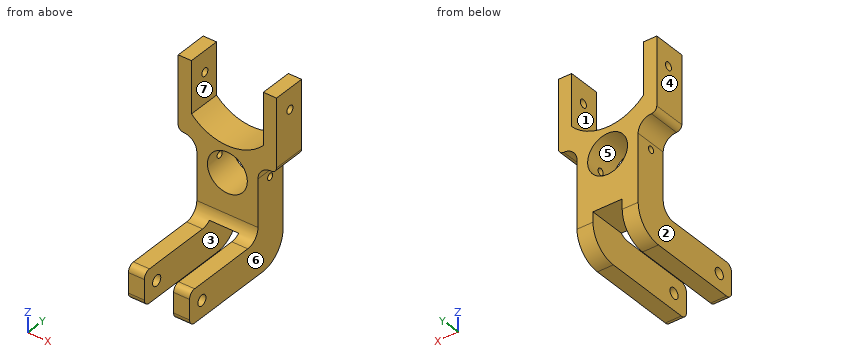
```python
from build123d import *

# Parameters (mm, degrees)
EXTRUDE_START         = -3
EXTRUDE_1_DEPTH       = 46
SKETCH_2_R            = 15
SKETCH_2_W            = 22
SKETCH_2_H            = 41.003909118
CUT_EXTRUDE_2_DEPTH   = 120
SKETCH_3_R            = 4
SKETCH_3_R_2          = 2.5
CUT_EXTRUDE_1_DEPTH   = 55
SKETCH_4_W            = 74
SKETCH_4_H            = 24.59688775
EXTRUDE_3_DEPTH       = 55
CUT_EXTRUDE_2_2_DEPTH = 50
FILLET_2_R            = 4
SKETCH_7_R            = 3
CUT_EXTRUDE_3_DEPTH   = 90
FILLET_3_R            = 10


with BuildPart() as part:
    # Эскиз1 → Вытянуть1 (new body)
    with BuildSketch(Plane(origin=(0, 0, 0), x_dir=(0, 0, -1), z_dir=(1, 0, 0)).offset(EXTRUDE_START)):
        with BuildLine():
            Line((3.683652722, 0), (3.683652722, -24.59688775))
            Line((3.683652722, -24.59688775), (49.132150834, -24.59688775))
            ThreePointArc((49.132150834, -24.59688775), (56.203219269, -27.52582056), (59.132150834, -34.59688951))
            Line((59.132150834, -34.59688951), (59.132141638, -86.831595085))
            ThreePointArc((59.132141638, -86.831595085), (60.596607421, -90.36712956), (64.132141638, -91.831595966))
            Line((64.132141638, -91.831595966), (79.132150834, -91.831595966))
            ThreePointArc((79.132150834, -91.831595966), (82.66768474, -90.367129871), (84.132150834, -86.831595966))
            Line((84.132150834, -86.831595966), (84.132150834, -20))
            ThreePointArc((84.132150834, -20), (78.274286458, -5.857864376), (64.132150834, 0))
            Line((64.132150834, 0), (3.683652722, 0))
        make_face()
    extrude(amount=EXTRUDE_1_DEPTH)

    # Эскиз2 → Cut-Extrude 2 (cut, symmetric)
    with BuildSketch(Plane(origin=(0, 0, 0), x_dir=(1, 0, 0), z_dir=(0, 1, 0))):
        with Locations(Location((20, 18.931682227, 0), (0, 0, 270))):
            Circle(SKETCH_2_R)
        with Locations((20, 77.079487522)):
            Rectangle(SKETCH_2_W, SKETCH_2_H)
    extrude(amount=CUT_EXTRUDE_2_DEPTH, both=True, mode=Mode.SUBTRACT)

    # Эскиз3 → Вырез-Вытянуть1 (cut, symmetric)
    with BuildSketch(Plane(origin=(0, 0, 0), x_dir=(0, 0, -1), z_dir=(1, 0, 0))):
        with Locations((71.632122158, -79.695359499)):
            Circle(SKETCH_3_R)
        with Locations((18.675004926, -12.628238718)):
            Circle(SKETCH_3_R_2)
    extrude(amount=CUT_EXTRUDE_1_DEPTH, both=True, mode=Mode.SUBTRACT)

    # Эскиз4 → Вытянуть3 (add)
    with BuildSketch(Plane.XY.offset(-3.683652722)):
        with Locations((20.003387868, -12.298443875)):
            Rectangle(SKETCH_4_W, SKETCH_4_H)
    extrude(amount=EXTRUDE_3_DEPTH)

    # Эскиз6 → Cut-Extrude 2 2 (cut, symmetric)
    with BuildSketch(Plane(origin=(0, 0, 0), x_dir=(1, 0, 0), z_dir=(0, 1, 0))):
        with BuildLine():
            Line((47.003387868, -53.712819086), (47.003387868, -12.467045061))
            ThreePointArc((47.003387868, -12.467045061), (20.003387863, -0.765266352), (-6.996612132, -12.467045083))
            Line((-6.996612132, -12.467045083), (-6.996612132, -53.712819086))
            Line((-6.996612132, -53.712819086), (47.003387868, -53.712819086))
        make_face()
    extrude(amount=CUT_EXTRUDE_2_2_DEPTH, both=True, mode=Mode.SUBTRACT)

    # Скругление2
    fillet_2_edges = [part.edges().sort_by_distance(p)[0] for p in [
        (57.003387868, -12.298443875, -3.683652722),
        (-16.996612132, -12.298443875, -3.683652722),
    ]]
    fillet(fillet_2_edges, radius=FILLET_2_R)

    # Эскиз7 → Вырез-Вытянуть3 (cut, symmetric)
    with BuildSketch(Plane(origin=(57.003387868, 0, 0), x_dir=(0, 0, -1), z_dir=(1, 0, 0))):
        with Locations((-35.623538585, -11.460561108)):
            Circle(SKETCH_7_R)
    extrude(amount=CUT_EXTRUDE_3_DEPTH, both=True, mode=Mode.SUBTRACT)

    # Скругление3
    fillet_3_edges = [part.edges().sort_by_distance(p)[0] for p in [
        (-3, -12.298443875, -3.683652722),
        (43, -12.298443875, -3.683652722),
    ]]
    fillet(fillet_3_edges, radius=FILLET_3_R)


solid = part.part
```
Geometry check sheet. Reference: the model listing, model coordinates, mm. Face numbers are marked on the shaded views. A direction names the side the tool comes from. Coordinates: 2 decimals unless noted, no trailing zeros. Order: outer loops, then holes, each group sorted by start corner. A loop starts at its lowest first (then second) coordinate and runs counter-clockwise, first axis right, second up. Notation, with made-up numbers: (-9.5, 15.25) - (34.5, 15.25) arc R21 ccw to (34.5, 46.25) - close; hole circle Ø8 at (61.5, -23). An arc over 180 degrees is marked (long way). Answer as a JSON object with one key per item and string values. Group by question number.
Item 1: Depth check by flat-ended pin: pin 1 Ø2 at (x, z) = (25, -43.5) entering from -Y; pin 2 Ø13 at (x, y) = (35.5, -71) entering from +Z; pin 3 Ø6 at (y, z) = (-79, -64.5) entering from +X. Enter the tip coordinate at first touch or a pass-through.
Item 2: Sectioned sample at B-B, the plane y = -60. Record the cut outline in (x, z), and give its area (3 significant figures).
Item 3: Draft check along X on the marked faces 4, 5, 6 and 7. Enter one of: +X half, -X half, draft (parallel to the pull), parting line (faces both ways), or undercut.
Item 4: Sectioned sample at C-C, the plane z = 15.5. Record the cut outline in (x, y).
Item 5: Scan lines: probe 1 along X at (y, z) = (-7, -76); probe 2 along X at (y, z) = (-12, 22); probe 3 along Z at (x, y) = (22.5, -24). Record each from-to range of solid material in increasing order.
Item 6: Sectioned sample at A-A, the plane x = 20. Record the cut outline in (y, z), and give its area (3 significant figures).
Item 7: Tool access check on the marked faces 1, 2 and 3. Record the directions out of +Z, -Z, +X, -X, +Y, -Y that give a thin tool (end or side, any length) a straight path to the whole face; none if there is none.
Resolved:
{
 "1": {"pin 1": "y = -24.6", "pin 2": "z = -59.13", "pin 3": "x = 43"},
 "2": {"outline": "(-3, -84.13) - (9, -84.13) - (9, -59.13) - (-3, -59.13) - close; (31, -84.13) - (43, -84.13) - (43, -59.13) - (31, -59.13) - close", "area": "600 mm^2"},
 "3": {"face 4": "-X half", "face 5": "undercut", "face 6": "+X half", "face 7": "undercut"},
 "4": {"outline": "(-17, -24.6) - (-7, -24.6) - (-7, 0) - (-17, 0) - close; (47, -24.6) - (57, -24.6) - (57, 0) - (47, 0) - close"},
 "5": {"probe 1": "-3 to 9, 31 to 43", "probe 2": "-17 to -7, 47 to 57", "probe 3": "-56.58 to -33.72, -4.14 to 0.85"},
 "6": {"outline": "(-27.92, -56.58) - (0, -56.58) - (0, -33.93) - (-24.6, -33.93) - (-24.6, -49.13) arc R10 cw to start; (-24.6, -3.93) - (0, -3.93) - (0, 0.77) - (-24.6, 0.77) - close", "area": "680 mm^2"},
 "7": {"face 1": "+Z, +Y, -Y", "face 2": "-Z, -X, +Y, -Y", "face 3": "-Z, +Y, -Y"}
}
